from build123d import *

# Parameters (mm, degrees)
SKETCH1_W           = 150
SKETCH1_H           = 150
BOSS_EXTRUDE1_DEPTH = 13
BOSS_EXTRUDE1_DRAFT = -45
SKETCH2_W           = 118
SKETCH2_H           = 59
CUT_EXTRUDE1_DEPTH  = 13


with BuildPart() as part:
    # Sketch1 → Boss-Extrude1 (with draft: the straight prism first)
    with BuildSketch(Plane(origin=(0, 0, 0), x_dir=(1, 0, 0), z_dir=(0, 1, 0))):
        with Locations((75, 75)):
            Rectangle(SKETCH1_W, SKETCH1_H)
    extrude(amount=BOSS_EXTRUDE1_DEPTH)
    # Boss-Extrude1: the draft: its side faces are tilted about the plane it starts from
    boss_extrude1_sides = [part.faces().sort_by_distance(p)[0] for p in [
        (75, 6.5, 0),
        (150, 6.5, -75),
        (75, 6.5, -150),
        (0, 6.5, -75),
    ]]
    draft(boss_extrude1_sides, Plane(origin=(0, 0, 0), x_dir=(1, 0, 0), z_dir=(0, 1, 0)), BOSS_EXTRUDE1_DRAFT)

    # Sketch2 → Cut-Extrude1 (cut)
    with BuildSketch(Plane(origin=(0, 13, 0), x_dir=(1, 0, 0), z_dir=(0, 1, 0))):
        with Locations((75, 43.5)):
            Rectangle(SKETCH2_W, SKETCH2_H)
    extrude(amount=-CUT_EXTRUDE1_DEPTH, mode=Mode.SUBTRACT)


solid = part.part
Geometry check sheet. Reference: the model listing, model coordinates, mm. A direction names the side the tool comes from. Round coordinates to 2 decimals unless told otherwise and drop trailing zeros. Order: outer loops, then holes, each group sorted by start corner. A loop starts at its lowest first (then second) coordinate and runs counter-clockwise, first axis right, second up. Notation, with made-up numbers: M 50.5,2 L 69.5,2 A17 cw 69.5,11 Z; hole C 89.5,66.25 d5. An arc over 180 degrees is marked long. Answer in a Markdown table with one row per item. Add a question column.
Item 1: Sectioned sample at A-A, the plane y = 7.5. Enter the section's corners in (x, z), plus the area to 3 significant figures.
Item 2: Draft check along Z on faces 1 (the face through (-6, 6, -74)), 2 (the face through (74, 6, -156)), 3 (the face through (134, 7, -43)). Enter one of: released by +Z, released by -Z, zero draft, split by the parting line, or undercut.
Item 3: Sectioned sample at D-D, the plane x = 147.5. Enter the section's corners in (y, z).
Item 4: Depth check by flat-ended pin: pin 1 Ø4 at (y, z) = (7, -74.5) entering from -X; pin 2 Ø4 at (y, z) = (7, -51.5) entering from +X; pin 3 Ø4 at (x, y) = (37.5, 6) entering from +Z. Enter the tip coordinate at first touch or a pass-through.
Item 5: Sectioned sample at B-B, the plane x = 67.5. Enter the section's corners in (y, z), plus the area to 3 significant figures.
Item 6: Set-up check for faces 4 (the face through (16, 7, -43)), 5 (the face through (74, 0, -93)): record each of +Z, -Z, +X, -X, +Y, -Y from which the full face is reachable in a straight line by a thin tool's end or side.
Item 7: Material ranges on L1, parallel to Z at x = 41, y = 5.75; L2, parallel to Z at x = 132, y = 5.5; L3, parallel to Z at x = 138.5, y = 7.5, recorded low to high. Write a range as [from, to].
Item 8: Sectioned sample at C-C, the plane z = -25.5. Enter the section's corners in (x, y).
Filled in:
| question | item | result |
|---|---|---|
| 1 | outline | M -7.5,-157.5 L 157.5,-157.5 L 157.5,7.5 L -7.5,7.5 Z; hole M 16,-73 L 134,-73 L 134,-14 L 16,-14 Z |
| 1 | area | 20,300 mm² |
| 2 | face 1 | zero draft |
| 2 | face 2 | released by -Z |
| 2 | face 3 | undercut |
| 3 | outline | M 0,-150 L 13,-163 L 13,13 L 0,0 Z |
| 4 | pin 1 | stops at x = -9 |
| 4 | pin 2 | stops at x = 159 |
| 4 | pin 3 | stops at z = 8 |
| 5 | outline | M 0,-150 L 13,-163 L 13,-73 L 0,-73 Z; M 0,-14 L 13,-14 L 13,13 L 0,0 Z |
| 5 | area | 1,350 mm² |
| 6 | face 4 | +Y, -Y |
| 6 | face 5 | +Z, -Z, +X, -X, -Y |
| 7 | L1 | z = [-155.75, -73], [-14, 5.75] |
| 7 | L2 | z = [-155.5, -73], [-14, 5.5] |
| 7 | L3 | z = [-157.5, 7.5] |
| 8 | outline | M -13,13 L 0,0 L 16,0 L 16,13 Z; M 134,0 L 150,0 L 163,13 L 134,13 Z |
